from build123d import *

# Parameters (mm, degrees)
BOSS_EXTRUDE2_DEPTH = 5
CUT_EXTRUDE1_START  = 5
SKETCH3_W           = 19.008841094
SKETCH3_H           = 2.1
SKETCH3_W_2         = 12
SKETCH3_W_3         = 1.535533906
SKETCH3_W_4         = 1.464466094
SKETCH3_W_5         = 17.544375
CUT_EXTRUDE1_DEPTH  = 16
CUT_EXTRUDE2_DEPTH  = 52
SKETCH5_W           = 1.05
SKETCH5_H           = 46.149322856
CUT_EXTRUDE3_DEPTH  = 10


with BuildPart() as part:
    # Sketch1 → Boss-Extrude2 (new body)
    with BuildSketch(Plane.XY):
        Polygon((-39.238867065, 47.72414844), (-47.72414844, 39.238867065), (-34.69381669, 26.208535316), (-26.208535316, 34.69381669), align=None)
        with BuildLine():
            ThreePointArc((-49.845468783, 62.573390845), (-56.568542495, 56.568542495), (-62.573390845, 49.845468783))
            Line((-62.573390845, 49.845468783), (-49.845468783, 37.117546722))
            Line((-49.845468783, 37.117546722), (-47.72414844, 39.238867065))
            Line((-47.72414844, 39.238867065), (-39.238867065, 47.72414844))
            Line((-39.238867065, 47.72414844), (-37.117546722, 49.845468783))
            Line((-37.117546722, 49.845468783), (-49.845468783, 62.573390845))
        make_face()
        with BuildLine():
            ThreePointArc((-34.594119865, 72.133534994), (-42.489529555, 67.783772971), (-49.845468783, 62.573390845))
            Line((-49.845468783, 62.573390845), (-37.117546722, 49.845468783))
            ThreePointArc((-37.117546722, 49.845468783), (-31.959737739, 60.548390845), (-34.594119865, 72.133534994))
        make_face()
        with BuildLine():
            ThreePointArc((-62.573390845, 49.845468783), (-67.783772971, 42.489529555), (-72.133534994, 34.594119865))
            ThreePointArc((-72.133534994, 34.594119865), (-60.548390845, 31.959737739), (-49.845468783, 37.117546722))
            Line((-49.845468783, 37.117546722), (-62.573390845, 49.845468783))
        make_face()
        with BuildLine():
            Line((-34.69381669, 26.208535316), (-35.779603128, 25.122748879))
            ThreePointArc((-35.779603128, 25.122748879), (-33.866185966, 25.503351216), (-32.244069222, 26.587214973))
            Line((-32.244069222, 26.587214973), (-26.587214973, 32.244069222))
            ThreePointArc((-26.587214973, 32.244069222), (-25.503351216, 33.866185966), (-25.122748879, 35.779603128))
            Line((-25.122748879, 35.779603128), (-26.208535316, 34.69381669))
            Line((-26.208535316, 34.69381669), (-34.69381669, 26.208535316))
        make_face()
    extrude(amount=BOSS_EXTRUDE2_DEPTH)

    # Sketch3 → Cut-Extrude1 (cut)
    with BuildSketch(Plane(origin=(-57.699913345, 57.699913345, 0), x_dir=(-0.707106781186549, -0.7071067811865461, 0), z_dir=(0.7071067811865461, -0.707106781186549, 0)).offset(CUT_EXTRUDE1_START)):
        with Locations((-17.039954453, -2.5)):
            Rectangle(SKETCH3_W, SKETCH3_H)
        with Locations((0, -2.5)):
            Rectangle(SKETCH3_W_2, SKETCH3_H)
        with Locations((-6.767766953, -2.5)):
            Rectangle(SKETCH3_W_3, SKETCH3_H)
        with Locations((6.767766953, -2.5)):
            Rectangle(SKETCH3_W_3, SKETCH3_H)
        with Locations((8.267766953, -2.5)):
            Rectangle(SKETCH3_W_4, SKETCH3_H)
        with Locations((17.7721875, -2.5)):
            Rectangle(SKETCH3_W_5, SKETCH3_H)
    extrude(amount=CUT_EXTRUDE1_DEPTH, mode=Mode.SUBTRACT)

    # Sketch4 → Cut-Extrude2 (cut)
    with BuildSketch(Plane(origin=(-57.699913345, 57.699913345, 0), x_dir=(-0.707106781186549, -0.7071067811865461, 0), z_dir=(0.7071067811865461, -0.707106781186549, 0))):
        Polygon((-7.535533906, -2.5), (27.054152634, -2.5), (27.054152634, -6.972921607), (-28.074504585, -6.972921607), (-28.074504585, -2.5), align=None)
    extrude(amount=CUT_EXTRUDE2_DEPTH, mode=Mode.SUBTRACT)

    # Sketch5 → Cut-Extrude3 (cut)
    with BuildSketch(Plane(origin=(-54.164379439, 54.164379439, 0), x_dir=(0, 0, -1), z_dir=(0.7071067811865461, -0.7071067811865489, 0))):
        with Locations((-1.975, 0)):
            Rectangle(SKETCH5_W, SKETCH5_H)
    extrude(amount=-CUT_EXTRUDE3_DEPTH, mode=Mode.SUBTRACT)


solid = part.part
For this review, take the finished solid that the model builds, in its own axes (mm). A direction names the side the tool comes from. Round coordinates to 2 decimals unless told otherwise and drop trailing zeros. Write each loop counter-clockwise with the first axis right and the second up, starting at its lowest first coordinate (ties: lowest second). Pieces come first, ordered by that corner, then holes. Notation, with made-up numbers: (7.25, 8) -> (28.25, 8) arc R17 cw to (28.25, 32) -> close; hole circle Ø11 at (-32, 85.5). An arc over 180 degrees is marked (long way). Put each result on its own line as item: value.
Q1. Consider section A-A on z = 0.85. State the section outline as (x, y) points.
Determined:
outline: (-72.13, 34.59) arc R18 ccw to (-49.85, 37.12) -> (-47.72, 39.24) -> (-34.69, 26.21) -> (-35.78, 25.12) arc R5 ccw to (-32.24, 26.59) -> (-26.59, 32.24) arc R5 ccw to (-25.12, 35.78) -> (-26.21, 34.69) -> (-39.24, 47.72) -> (-37.12, 49.85) arc R18 ccw to (-34.59, 72.13) arc R80 ccw to start
Q2. Consider section C-C on x = -42. State the section outline as (y, z) points.
Determined:
outline: (33.51, 0) -> (68.09, 0) -> (68.09, 1.45) -> (43.7, 1.45) -> (43.7, 2.5) -> (33.51, 2.5) -> close
Q3. Consider section B-B on y = 41. State the section outline as (x, z) points.
Determined:
outline: (-68.69, 0) -> (-32.51, 0) -> (-32.51, 2.5) -> (-44.7, 2.5) -> (-44.7, 1.45) -> (-68.69, 1.45) -> close
Q4. The part is to be moulded in two halves that separate along X. For faces 1 (the cylindrical face through (-31.98, 60.38, 0.71)), 2 (the flat face through (-25.7, 35.2, 1.2)), 3 (the flat face through (-36, 36, 2.5)), say which applies: released by +X, released by -X, zero draft, split by the parting line, or undercut.
Determined:
face 1: released by +X
face 2: undercut
face 3: zero draft
Q5. Machinability: for faces 4 (the flat face through (-42.8, 42.9, 2)), 5 (the flat face through (-48.8, 38.163, 0.715)), 6 (the flat face through (-35.2, 25.7, 1.2)), which of the approach directions +Z, -Z, +X, -X, +Y, -Y give a long, thin tool a straight path to every point of the face, cutting with its end or side? Answer none if there is none.
Determined:
face 4: +Z, -X, +Y
face 5: +Z, -Z, -Y
face 6: +Z, -Z, -X
Q6. Consider section D-D on x = -56. State the section outline as (y, z) points.
Determined:
outline: (33.09, 0) -> (57.13, 0) -> (57.13, 1.45) -> (33.09, 1.45) -> close
Q7. Clearance check with flat-ended pins moving along their axes: pin 1 Ø3 at (x, y) = (-53.5, 39.5) entering from +Z; pin 2 Ø1.5 at (x, y) = (-50, 34.5) entering from +Z; pin 3 Ø1 at (x, z) = (-49.5, 1) entering from -Y. State where each tip first meets the part, or that it passes through.
Determined:
pin 1: stops at z = 1.45
pin 2: passes through
pin 3: stops at y = 36.96
Q8. To check wall thickness, follow L1, parallel to Y at x = -35, z = 0.5; L2, parallel to Z at x = -47, y = 51.5. State the ranges of each line that lie inside material, in increasing order. Write a range as [from, to].
Determined:
L1: y = [25.18, 25.9], [26.51, 43.49], [52.39, 71.94]
L2: z = [0, 1.45]
